from build123d import *

# Parameters (mm, degrees)
CLAMP_BAR_SKETCH_W       = 32
CLAMP_BAR_SKETCH_H       = 118
CLAMP_BAR_DEPTH          = 2
FINGER_RELIEF_SKETCH_W   = 10.4
FINGER_RELIEF_SKETCH_H   = 12.3
FINGER_RELIEFS_DEPTH     = 2.4
FOLDED_FINGERS_DEPTH     = 10
STUD_CLEARANCES_SKETCH_R = 3.3
STUD_CLEARANCES_DEPTH    = 2.4


with BuildPart() as part:
    # Clamp Bar Sketch → Clamp Bar (new body)
    with BuildSketch(Plane.XY.offset(140)):
        with Locations((-7.5, 0)):
            Rectangle(CLAMP_BAR_SKETCH_W, CLAMP_BAR_SKETCH_H)
    extrude(amount=CLAMP_BAR_DEPTH)

    # Finger Relief Sketch → Finger Reliefs (cut)
    with BuildSketch(Plane.XY.offset(139.8)):
        with Locations((-7.5, -50.15)):
            Rectangle(FINGER_RELIEF_SKETCH_W, FINGER_RELIEF_SKETCH_H)
        with Locations((-7.5, 50.15)):
            Rectangle(FINGER_RELIEF_SKETCH_W, FINGER_RELIEF_SKETCH_H)
    extrude(amount=FINGER_RELIEFS_DEPTH, mode=Mode.SUBTRACT)

    # Folded Finger Sketch → Folded Fingers (add)
    with BuildSketch(Plane(origin=(-12.5, 0, 0), x_dir=(0, 0, -1), z_dir=(1, 0, 0))):
        with BuildLine():
            Line((-138, -48), (-130, -48))
            Line((-130, -48), (-130, -46))
            Line((-130, -46), (-138, -46))
            ThreePointArc((-138, -46), (-139.414213562, -45.414213562), (-140, -44))
            Line((-140, -44), (-142, -44))
            ThreePointArc((-142, -44), (-140.828427125, -46.828427125), (-138, -48))
        make_face()
        with BuildLine():
            Line((-138, 48), (-130, 48))
            Line((-130, 48), (-130, 46))
            Line((-130, 46), (-138, 46))
            ThreePointArc((-138, 46), (-139.414213562, 45.414213562), (-140, 44))
            Line((-140, 44), (-142, 44))
            ThreePointArc((-142, 44), (-140.828427125, 46.828427125), (-138, 48))
        make_face()
    extrude(amount=FOLDED_FINGERS_DEPTH)

    # Stud Clearances Sketch → Stud Clearances (cut)
    with BuildSketch(Plane.XY.offset(139.8)):
        with Locations((-18, -51.5)):
            Circle(STUD_CLEARANCES_SKETCH_R)
        with Locations((-18, 51.5)):
            Circle(STUD_CLEARANCES_SKETCH_R)
    extrude(amount=STUD_CLEARANCES_DEPTH, mode=Mode.SUBTRACT)


solid = part.part
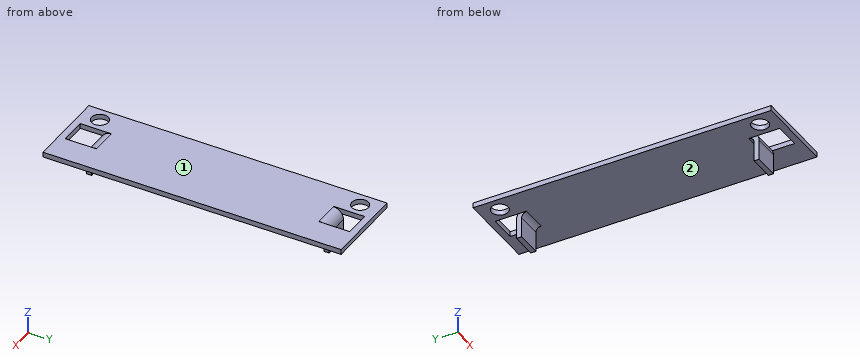
Model file for the job. Use its own axes, mm. Face numbers are marked on the shaded views. Give positions to 0.01 mm unless a question says otherwise; leave off trailing zeros. Loops run counter-clockwise (first coordinate to the right, second up) from the corner with the lowest first, then second, coordinate; pieces in that order, holes last.
1) Wall check: line 1 (X direction, y = -51.5, z = 140.8); line 2 (Y direction, x = -18, z = 140.65); line 3 (Y direction, x = -9, z = 131.5). Give the ranges that are in metal, low to high.
2) Saw through at A-A (x = -5.5). Write the cut outline in (y, z).
3) Pull direction Y, two halves, no side cores. Call the marked faces 1 and 2: +Y half, -Y half, draft (parallel to the pull), parting line (faces both ways), or undercut.
4) Flat gauge pins, fed straight in: pin 1 Ø4 at (x, z) = (-7.5, 134.5) entering from -Y; pin 2 Ø4.5 at (y, z) = (46, 138) entering from -X; pin 3 Ø1.2 at (y, z) = (-46.5, 138) entering from -X; pin 4 Ø4 at (x, z) = (-8.5, 132.5) entering from +Y. Where does each tip first touch, or does it go through?
5) Saw through at D-D (x = -0.5). Write the cut outline in (y, z), plus the area to 3 significant figures.
6) Saw through at B-B (y = -51.5). Write the cut outline in (x, z).
7) Saw through at C-C (z = 132.75). Write the cut outline in (x, y), plus the area to 3 significant figures.
Answer block:
1. line 1: x = -23.5 to -21.3, -14.7 to -12.7, -2.3 to 8.5
1. line 2: y = -59 to -54.8, -48.2 to 48.2, 54.8 to 59
1. line 3: y = -48 to -46, 46 to 48
2. outline: (-59, 140) - (-56.3, 140) - (-56.3, 142) - (-59, 142) - close; (-48, 130) - (-46, 130) - (-46, 138) arc R2 cw to (-44, 140) - (44, 140) arc R2 cw to (46, 138) - (46, 130) - (48, 130) - (48, 138) arc R4 ccw to (44, 142) - (-44, 142) arc R4 ccw to (-48, 138) - close; (56.3, 140) - (59, 140) - (59, 142) - (56.3, 142) - close
3. face 1: draft
3. face 2: undercut
4. pin 1: stops at y = -48
4. pin 2: stops at x = -23.5
4. pin 3: stops at x = -12.5
4. pin 4: stops at y = 48
5. outline: (-59, 140) - (59, 140) - (59, 142) - (-59, 142) - close
5. area: 236 mm2
6. outline: (-23.5, 140) - (-21.3, 140) - (-21.3, 142) - (-23.5, 142) - close; (-14.7, 140) - (-12.7, 140) - (-12.7, 142) - (-14.7, 142) - close; (-2.3, 140) - (8.5, 140) - (8.5, 142) - (-2.3, 142) - close
7. outline: (-12.5, -48) - (-2.5, -48) - (-2.5, -46) - (-12.5, -46) - close; (-12.5, 46) - (-2.5, 46) - (-2.5, 48) - (-12.5, 48) - close
7. area: 40.0 mm2
